```python
from build123d import *

# Parameters (mm, degrees)
PAD017_DEPTH           = 5
PAD020_DEPTH           = 6.25
SKETCH040_W            = 5.2
SKETCH040_H            = 1.65
PAD022_DEPTH           = 2.1
SKETCH041_W            = 2.1
SKETCH041_H            = 1.65
PAD023_DEPTH           = 5
SKETCH042_W            = 5.2
SKETCH042_H            = 1.65
PAD024_DEPTH           = 5
LINEARPATTERN010_COUNT = 2
LINEARPATTERN010_PITCH = 3.3
CHAMFER_SIZE           = 1


with BuildPart() as obj1:
    # Sketch034 → Pad017 (new body)
    with BuildSketch(Plane.XY):
        with BuildLine():
            Line((-1.35, -1.8), (-1.35, 6))
            ThreePointArc((0, 7.35), (-0.954594, 6.954594), (-1.35, 6))
            Line((0, 9), (0, 7.35))
            Line((-2.6, 9), (0, 9))
            Line((-2.6, -1.8), (-2.6, 9))
            Line((-3.85, -1.8), (-2.6, -1.8))
            ThreePointArc((-3.85, -1.8), (-3.439949, -2.789949), (-2.45, -3.2))
            Line((-1.35, -3.2), (-2.45, -3.2))
            Line((-1.35, -1.8), (-1.35, -3.2))
        make_face()
    extrude(amount=PAD017_DEPTH)

    # Sketch037 → Pad020 (join)
    with BuildSketch(Plane.XY):
        Polygon((-1.35, 0.2), (-1.35, 1.6), (-2.6, 1.6), (-3.85, 1.6), (-3, 0.2), (-2.6, 0.2), align=None)
    extrude(amount=PAD020_DEPTH)


with BuildPart() as obj2:
    # Mirror001: instance of _obj1
    add(obj1.part.mirror(Plane(origin=(0, 0, 0), x_dir=(0, 1, 0), z_dir=(-1, 0, 0))))


with BuildPart() as body012:
    # Fusion001 base: copy of _obj1
    add(obj1.part)

    # Fusion001: union _obj2)
    add(obj2.part)

    # Sketch040 → Pad022 (new body)
    with BuildSketch(Plane.XY):
        with Locations((0, 9.825)):
            Rectangle(SKETCH040_W, SKETCH040_H)
    pad022 = extrude(amount=PAD022_DEPTH)

    # Sketch041 → Pad023 (join)
    with BuildSketch(Plane.XY):
        with Locations((1.55, 9.825)):
            Rectangle(SKETCH041_W, SKETCH041_H)
    pad023 = extrude(amount=PAD023_DEPTH)

    # Sketch042 → Pad024 (join)
    with BuildSketch(Plane.XY):
        with Locations((0, 11.475)):
            Rectangle(SKETCH042_W, SKETCH042_H)
    pad024 = extrude(amount=PAD024_DEPTH)

    # LinearPattern010: Pad024, Pad023, Pad022 ×2
    with Locations(*[(0, i * LINEARPATTERN010_PITCH, 0) for i in range(1, LINEARPATTERN010_COUNT)]):
        add(pad024)
        add(pad023)
        add(pad022)

    # Chamfer
    chamfer_edges = [body012.edges().sort_by_distance(p)[0] for p in [
        (-2.6, 5.3, 5),
        (-2.6, 11.475, 5),
        (-2.6, 14.775, 5),
    ]]
    chamfer(chamfer_edges, length=CHAMFER_SIZE)


solid = body012.part
```
Geometry: final body of the model. Coordinates: model frame, mm. A direction names the side the tool comes from. Round coordinates to 2 decimals unless told otherwise and drop trailing zeros. Write each loop counter-clockwise with the first axis right and the second up, starting at its lowest first coordinate (ties: lowest second). Pieces come first, ordered by that corner, then holes. Notation, with made-up numbers: (83.5, -11.75) -> (98.5, -11.75) arc R27 ccw to (98.5, 18.25) -> close; hole circle Ø8 at (-31.5, 63). An arc over 180 degrees is marked (long way). Use CSV: the item, a comma, the result in double quotes. Start each with the question number.
Q1. First-contact query: pin 1 Ø1 at (y, z) = (-1, 2) entering from -X; pin 2 Ø0.6 at (x, z) = (-3.5, 2.5) entering from +Y; pin 3 Ø1 at (x, y) = (-0.5, 5) entering from -Z; pin 4 Ø0.8 at (x, y) = (-2, -2) entering from +Z. Flat tips, straight axial feed; report the tip coordinate or a pass-through.
Q2. Section C-C (x = 2). Return loops of the section in (y, z), plus the area to 4 significant figures.
Q3. Reachability of faces 4 (the face through (2.6, -1, 2)), 5 (the face through (-3, -1.8, 2)), 6 (the face through (1, 10, 5)), 7 (the face through (-1, 10, 2.1)) from +Z, -Z, +X, -X, +Y, -Y: full face, straight path, thin tool, end or side. Return the list, or none.
Q4. Section A-A (y = 3). Return loops of the section in (x, z), plus the area to 3 significant figures.
Q5. Pull-direction query (X, two-part tool) for faces 1 (the face through (3.45, -2.78, 2.46)), 2 (the face through (-1.35, 1, 2)), 3 (the face through (-1, 12.3, 4)); classes: pulls with the +X half, pulls with the -X half, needs draft (parallel to the pull), parting line crosses it, or undercut.
Q6. Section B-B (z = 5.5). Return loops of the section in (x, y), plus the area to 3 significant figures.
Q7. Line query: L1, parallel to Y at x = -2.25, z = 2.5; L2, parallel to X at y = -0.75, z = 3.25; L3, parallel to X at y = 9.5, z = 3.5. Output: solid intervals per line, ascending.
Result sheet:
1,pin 1,"x = -2.6"
1,pin 2,"y = 1.6"
1,pin 3,"through"
1,pin 4,"z = 5"
2,outline,"(-3.2, 0) -> (15.6, 0) -> (15.6, 5) -> (1.6, 5) -> (1.6, 6.25) -> (0.2, 6.25) -> (0.2, 5) -> (-3.2, 5) -> close"
2,area,"95.75 mm²"
3,face 4,"+Z, -Z, +X"
3,face 5,"+Z, -Z, -X"
3,face 6,"+Z, +X, -X, +Y"
3,face 7,"+Z, -X"
4,outline,"(-2.6, 0) -> (-1.35, 0) -> (-1.35, 5) -> (-1.6, 5) -> (-2.6, 4) -> close; (1.35, 0) -> (2.6, 0) -> (2.6, 5) -> (1.35, 5) -> close"
4,area,"12.0 mm²"
5,face 1,"pulls with the +X half"
5,face 2,"undercut"
5,face 3,"needs draft"
6,outline,"(-3.85, 1.6) -> (-3, 0.2) -> (-1.35, 0.2) -> (-1.35, 1.6) -> close; (1.35, 0.2) -> (3, 0.2) -> (3.85, 1.6) -> (1.35, 1.6) -> close"
6,area,"5.81 mm²"
7,L1,"-3.2 to 9, 10.65 to 12.3, 13.95 to 15.6"
7,L2,"-2.6 to -1.35, 1.35 to 2.6"
7,L3,"0.5 to 2.6"
